Verification items for the finished model (mm, model axes). A direction names the side the tool comes from. Coordinates: 2 decimals unless noted, no trailing zeros. Order: outer loops, then holes, each group sorted by start corner. A loop starts at its lowest first (then second) coordinate and runs counter-clockwise, first axis right, second up. Notation, with made-up numbers: (75, 73) -> (112, 73) arc R10 cw to (112, 91) -> close; hole circle Ø9 at (-19, 52). An arc over 180 degrees is marked (long way). Write item = value, one per line. Start each with the question number.
1. Go/stop test with flat-tipped pins: P1, Ø2, axis at y = -13, z = 7, coming from the +X side; P2, Ø8, axis at y = -7, z = 7, coming from the -X side; P3, Ø5, axis at x = 10, z = 12, coming from the +Y side. Record where each tip stops, or that it passes through.
2. Release check for a two-part mould opening along Y. For faces 4 (the cylindrical face through (13.38, -25.73, 7.89)), 5 (the cylindrical face through (23.846, 7.509, 7.888)), 6 (the flat face through (13, 22, 16)) record: +Y half, -Y half, draft (parallel to the pull), parting line (faces both ways), or undercut.
3. Cross-section at A-A on x = -20. Record the cut outline in (y, z), plus the area to 3 significant figures.
4. Cross-section at B-B on x = 0. Record the cut outline in (y, z).
5. Set-up check for faces 1 (the flat face through (13, 22, 0)), 2 (the cylindrical face through (-1.774, 26.989, 3.032)), 3 (the cylindrical face through (0, -27, 15)): record each of +Z, -Z, +X, -X, +Y, -Y from which the full face is reachable in a straight line by a thin tool's end or side.
6. Cross-section at C-C on y = 0. Record the cut outline in (x, z).
7. Thickness scan on line 1 along Y through (x, z) = (0, 6.5); line 2 along Y through (x, z) = (-20, 11.25); line 3 along X through (y, z) = (7, 6.5). Record the ranges inside material, lowest first. Write a range as from..to.
8. Cross-section at D-D on z = 13. Record the cut outline in (x, y).
from build123d import *

# Parameters (mm, degrees)
SKETCH1_R           = 29
SKETCH1_R_2         = 25
BOSS_EXTRUDE1_DEPTH = 16
SKETCH3_R           = 2
CUT_EXTRUDE1_DEPTH  = 16
SKETCH4_R           = 2
CUT_EXTRUDE2_DEPTH  = 16


with BuildPart() as part:
    # Sketch1 → Boss-Extrude1 (new body)
    with BuildSketch(Plane.XY):
        Circle(SKETCH1_R)
        Circle(SKETCH1_R_2, mode=Mode.SUBTRACT)
    extrude(amount=BOSS_EXTRUDE1_DEPTH)

    # Sketch3 → Cut-Extrude1 (cut)
    with BuildSketch(Plane(origin=(0, 29, 0), x_dir=(1, 0, 0), z_dir=(0, 1, 0))):
        with Locations(Location((0, -2.108912796, 0), (0, 0, 270))):
            Circle(SKETCH3_R)
    extrude(amount=-CUT_EXTRUDE1_DEPTH, mode=Mode.SUBTRACT)

    # Sketch4 → Cut-Extrude2 (cut)
    with BuildSketch(Plane(origin=(0, -29, 0), x_dir=(1, 0, 0), z_dir=(0, 1, 0))):
        with Locations(Location((0, -13, 0), (0, 0, 90))):
            Circle(SKETCH4_R)
    extrude(amount=CUT_EXTRUDE2_DEPTH, mode=Mode.SUBTRACT)


solid = part.part
Worked out:
q1.P1 = 26.4
q1.P2 = -28.84
q1.P3 = 28.01
q2.face_4 = parting line
q2.face_5 = undercut
q2.face_6 = draft
q3.outline = (-21, 0) -> (-15, 0) -> (-15, 16) -> (-21, 16) -> close; (15, 0) -> (21, 0) -> (21, 16) -> (15, 16) -> close
q3.area = 192 mm²
q4.outline = (-29, 0) -> (-25, 0) -> (-25, 11) -> (-29, 11) -> close; (-29, 15) -> (-25, 15) -> (-25, 16) -> (-29, 16) -> close; (25, 0) -> (29, 0) -> (29, 0.11) -> (25, 0.11) -> close; (25, 4.11) -> (29, 4.11) -> (29, 16) -> (25, 16) -> close
q5.face_1 = -Z, +X, -X, +Y, -Y
q5.face_2 = +Y
q5.face_3 = -Y
q6.outline = (-29, 0) -> (-25, 0) -> (-25, 16) -> (-29, 16) -> close; (25, 0) -> (29, 0) -> (29, 16) -> (25, 16) -> close
q7.line_1 = -29..-25, 25..29
q7.line_2 = -21..-15, 15..21
q7.line_3 = -28.14..-24, 24..28.14
q8.outline = (-2, -28.93) -> (-2, -24.92) arc R25 cw (long way) to (2, -24.92) -> (2, -28.93) arc R29 ccw (long way) to start
